Check sheet for the drawn part. Datum: minimum x, y, z corner. Units: mm. A direction names the side the tool comes from. Coordinates: 2 decimals unless noted, no trailing zeros. Write each loop counter-clockwise with the first axis right and the second up, starting at its lowest first coordinate (ties: lowest second). Pieces come first, ordered by that corner, then holes. Notation, with made-up numbers: (84, 19) -> (100, 19) arc R25 ccw to (100, 42) -> close; hole circle Ø3 at (30, 36). An arc over 180 degrees is marked (long way). Answer in a Markdown table with one row per item.
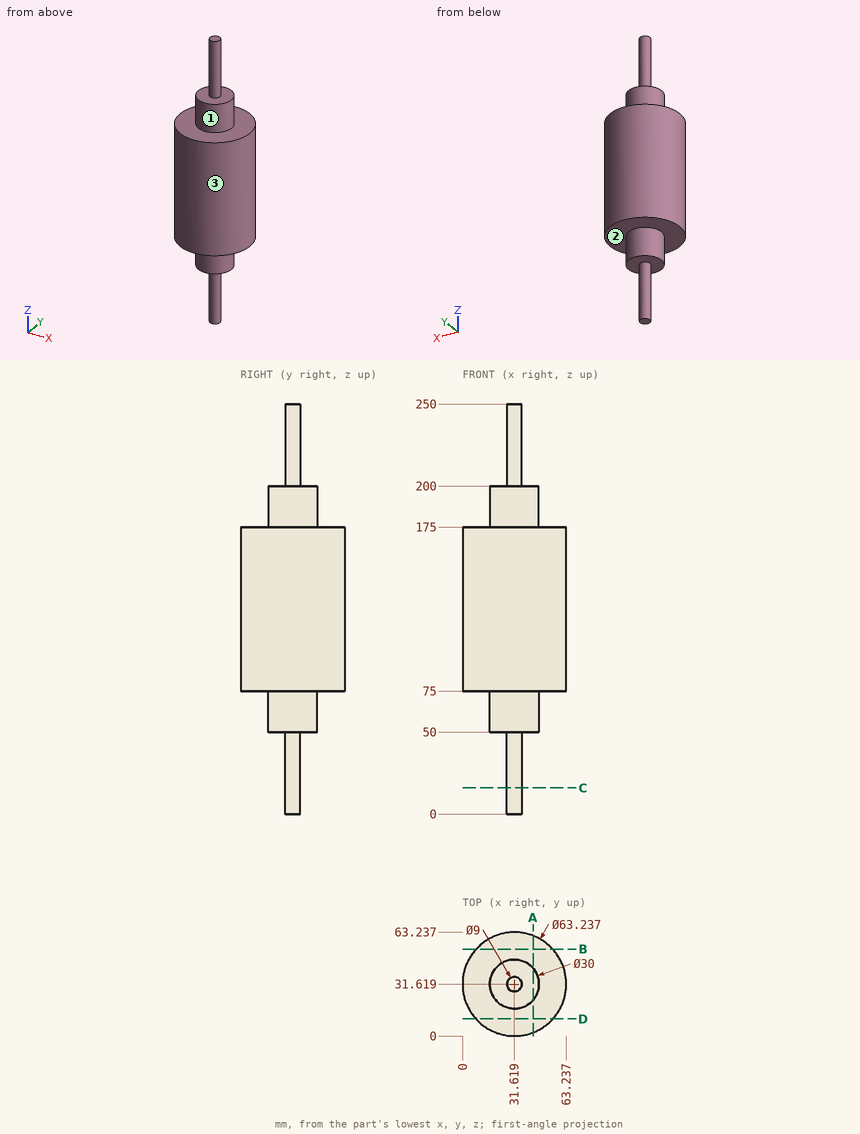
1. Sectioned sample at B-B, the plane y = 53. Record the cut outline in (x, z) (1 decimal).
Findings below:
| item | result |
|---|---|
| outline | (8.3, 75) -> (54.9, 75) -> (54.9, 175) -> (8.3, 175) -> close |
2. Sectioned sample at A-A, the plane x = 43. Record the cut outline in (y, z).
Findings below:
| item | result |
|---|---|
| outline | (2.12, 75) -> (21.85, 75) -> (21.85, 50) -> (41.39, 50) -> (41.39, 75) -> (61.12, 75) -> (61.12, 175) -> (41.39, 175) -> (41.39, 200) -> (21.85, 200) -> (21.85, 175) -> (2.12, 175) -> close |
3. Sectioned sample at C-C, the plane z = 16. Record the cut outline in (x, y), and give its area (3 significant figures).
Findings below:
| item | result |
|---|---|
| outline | circle Ø9 at (31.62, 31.62) |
| area | 63.6 mm² |
4. Sectioned sample at D-D, the plane y = 10.5. Record the cut outline in (x, z).
Findings below:
| item | result |
|---|---|
| outline | (8.09, 75) -> (55.15, 75) -> (55.15, 175) -> (8.09, 175) -> close |
5. Material ranges on probe 1 along Z at (x, y) = (37, 40.5); probe 2 along Z at (x, y) = (30, 15); probe 3 along X at (y, z) = (29, 122.5), recorded low to high. Write a range as from..to.
Findings below:
| item | result |
|---|---|
| probe 1 | z = 50..200 |
| probe 2 | z = 75..175 |
| probe 3 | x = 0.11..63.13 |
6. Access from +Z, -Z, +X, -X, +Y, -Y to the whole of each face (thin tool, end or side, straight path). Record for the marked faces 1, 2 and 3.
Findings below:
| item | result |
|---|---|
| face 1 | +Z |
| face 2 | -Z |
| face 3 | +Z, -Z |
7. Go/stop test with flat-tipped pins: pin 1 (8 mm diameter, centred on x = 34.5, z = 74, fed in from -Y); pin 2 (19 mm diameter, centred on x = 38.5, y = 28.5, fed in from -Z); pin 3 (2 mm diameter, centred on x = 21, y = 40, fed in from -Z); pin 4 (10 mm diameter, centred on x = 7, z = 134.5, fed in from +Y) (1 decimal). Record where each tip stops, or that it passes through.
Findings below:
| item | result |
|---|---|
| pin 1 | stops at y = 0 |
| pin 2 | stops at z = 0 |
| pin 3 | stops at z = 50 |
| pin 4 | stops at y = 56.4 |
